```python
from build123d import *

# Parameters (mm, degrees)
PAD006_DEPTH    = 5.1
PAD007_DEPTH    = 2
SKETCH012_W     = 19.5
SKETCH012_H     = 3.5
POCKET004_DEPTH = 26
POCKET005_DEPTH = 5
SKETCH014_R     = 0.575
POCKET006_DEPTH = 3.6
SKETCH015_R     = 1
POCKET007_DEPTH = 2
SKETCH016_W     = 4.5
SKETCH016_H     = 1
PAD008_DEPTH    = 1
CHAMFER_SIZE    = 0.99
SKETCH017_W     = 4.5
SKETCH017_H     = 1
PAD009_DEPTH    = 1
CHAMFER001_SIZE = 0.99
SKETCH018_W     = 9.5
SKETCH018_H     = 10
POCKET008_DEPTH = 4.4
SKETCH022_W     = 4.5
SKETCH022_H     = 1
PAD011_DEPTH    = 1
CHAMFER002_SIZE = 0.99
SKETCH023_W     = 10
SKETCH023_H     = 23.75
PAD012_DEPTH    = 5.1


with BuildPart() as part:
    # Sketch010 → Pad006 (new body)
    with BuildSketch(Plane.XY.offset(7.4)):
        with BuildLine():
            Line((149.259997, 103.29), (149.259997, 4))
            ThreePointArc((145.259999, 0), (148.088425, 1.171573), (149.259997, 4))
            Line((3.999999, 0), (145.259999, 0))
            ThreePointArc((0, 4), (1.171572, 1.171573), (3.999999, 0))
            Line((0, 103.29), (0, 4))
            ThreePointArc((3.999997, 107.29), (1.171572, 106.118426), (0, 103.29))
            Line((3.999997, 107.29), (145.259997, 107.29))
            ThreePointArc((149.259997, 103.29), (148.088425, 106.118427), (145.259997, 107.29))
        make_face()
        with BuildLine():
            Line((3.999997, 105.69), (145.259997, 105.69))
            ThreePointArc((147.659997, 103.29), (146.957054, 104.987056), (145.259997, 105.69))
            Line((147.659997, 103.29), (147.659997, 4))
            ThreePointArc((145.259999, 1.6), (146.957054, 2.302944), (147.659997, 4))
            Line((66.05, 1.6), (145.259999, 1.6))
            Line((66.05, 1.6), (66.05, 25.35))
            Line((66.05, 25.35), (38.05, 25.35))
            Line((38.05, 25.35), (38.05, 1.6))
            Line((4, 1.6), (38.05, 1.6))
            ThreePointArc((1.6, 4), (2.302944, 2.302944), (4, 1.6))
            Line((1.6, 103.29), (1.6, 4))
            ThreePointArc((3.999997, 105.69), (2.302943, 104.987055), (1.6, 103.29))
        make_face(mode=Mode.SUBTRACT)
    extrude(amount=PAD006_DEPTH)

    # Sketch011 (on Face22 of Pad006) → Pad007 (join)
    with BuildSketch(Plane.XY.offset(12.5)):
        with BuildLine():
            Line((149.259997, 103.29), (149.259997, 4))
            ThreePointArc((145.259999, 0), (148.088425, 1.171573), (149.259997, 4))
            Line((3.999999, 0), (145.259999, 0))
            ThreePointArc((0, 4), (1.171572, 1.171573), (3.999999, 0))
            Line((0, 103.29), (0, 4))
            ThreePointArc((3.999997, 107.29), (1.171572, 106.118426), (0, 103.29))
            Line((3.999997, 107.29), (145.259997, 107.29))
            ThreePointArc((149.259997, 103.29), (148.088425, 106.118427), (145.259997, 107.29))
        make_face()
        Polygon((8.05, 102.19), (8.05, 7.1), (28.05, 7.1), (28.05, 25.35), (66.05, 25.35), (66.05, 7.1), (141.209997, 7.1), (141.209997, 83.13), (122.759997, 83.13), (122.759997, 102.19), align=None, mode=Mode.SUBTRACT)
    extrude(amount=PAD007_DEPTH)

    # Sketch012 (on Face26 of Pad007) → Pocket004 (cut)
    with BuildSketch(Plane.YZ.offset(66.05)):
        with Locations((13.3, 9.15)):
            Rectangle(SKETCH012_W, SKETCH012_H)
    extrude(amount=-POCKET004_DEPTH, mode=Mode.SUBTRACT)

    # Sketch013 (on Face25 of Pocket004) → Pocket005 (cut)
    with BuildSketch(Plane.XY.offset(14.5)):
        with BuildLine():
            ThreePointArc((45.3, 15.325), (42.8, 12.825), (45.3, 10.325))
            Line((45.3, 10.325), (46.8, 10.325))
            ThreePointArc((46.8, 10.325), (49.3, 12.825), (46.8, 15.325))
            Line((45.3, 15.325), (46.8, 15.325))
        make_face()
    extrude(amount=-POCKET005_DEPTH, mode=Mode.SUBTRACT)

    # Sketch014 (on Face29 of Pocket005) → Pocket006 (cut)
    with BuildSketch(Plane(origin=(0, 0, 10.9), x_dir=(1, 0, 0), z_dir=(0, 0, -1))):
        with Locations((56.8, -7.825)):
            Circle(SKETCH014_R)
        with Locations((56.8, -17.825)):
            Circle(SKETCH014_R)
    extrude(amount=-POCKET006_DEPTH, mode=Mode.SUBTRACT)

    # Sketch015 (on Face29 of Pocket006) → Pocket007 (cut)
    with BuildSketch(Plane(origin=(0, 0, 10.9), x_dir=(1, 0, 0), z_dir=(0, 0, -1))):
        with Locations((56.8, -17.825)):
            Circle(SKETCH015_R)
        with Locations((56.8, -7.825)):
            Circle(SKETCH015_R)
    extrude(amount=-POCKET007_DEPTH, mode=Mode.SUBTRACT)

    # Sketch016 (on Face6 of Pocket007) → Pad008 (join)
    with BuildSketch(Plane.YZ.offset(147.659997)):
        with Locations((11.3, 7.9)):
            Rectangle(SKETCH016_W, SKETCH016_H)
        with Locations((95.99, 7.9)):
            Rectangle(SKETCH016_W, SKETCH016_H)
    extrude(amount=-PAD008_DEPTH)

    # Chamfer
    chamfer_edges = [part.edges().sort_by_distance(p)[0] for p in [
        (146.659997, 11.3, 7.4),
        (146.659997, 95.99, 7.4),
    ]]
    chamfer(chamfer_edges, length=CHAMFER_SIZE)

    # Sketch017 (on Face31 of Chamfer) → Pad009 (join)
    with BuildSketch(Plane(origin=(1.6, 0, 0), x_dir=(0, -1, 0), z_dir=(-1, 0, 0))):
        with Locations((-95.99, 7.9)):
            Rectangle(SKETCH017_W, SKETCH017_H)
        with Locations((-11.3, 7.9)):
            Rectangle(SKETCH017_W, SKETCH017_H)
    extrude(amount=-PAD009_DEPTH)

    # Chamfer001
    chamfer001_edges = [part.edges().sort_by_distance(p)[0] for p in [
        (2.6, 95.99, 7.4),
        (2.6, 11.3, 7.4),
    ]]
    chamfer(chamfer001_edges, length=CHAMFER001_SIZE)

    # Sketch018 (on Face47 of Chamfer001) → Pocket008 (cut)
    with BuildSketch(Plane.XY.offset(14.5)):
        with Locations((133.009997, 102.29)):
            Rectangle(SKETCH018_W, SKETCH018_H)
    extrude(amount=-POCKET008_DEPTH, mode=Mode.SUBTRACT)

    # Sketch022 (on Face31 of Pocket008) → Pad011 (join)
    with BuildSketch(Plane(origin=(0, 105.69, 0), x_dir=(-1, 0, 0), z_dir=(0, 1, 0))):
        with Locations((-111.959997, 7.9)):
            Rectangle(SKETCH022_W, SKETCH022_H)
    extrude(amount=-PAD011_DEPTH)

    # Chamfer002
    chamfer002_edges = [part.edges().sort_by_distance(p)[0] for p in [
        (111.959997, 104.69, 7.4),
    ]]
    chamfer(chamfer002_edges, length=CHAMFER002_SIZE)

    # Sketch023 (on Face42 of Chamfer002) → Pad012 (join)
    with BuildSketch(Plane(origin=(0, 0, 12.5), x_dir=(1, 0, 0), z_dir=(0, 0, -1))):
        with Locations((33.05, -13.475)):
            Rectangle(SKETCH023_W, SKETCH023_H)
    extrude(amount=PAD012_DEPTH)


solid = part.part
```
For this review, take the finished solid that the model builds, in its own axes (mm). A direction names the side the tool comes from. Round coordinates to 2 decimals unless told otherwise and drop trailing zeros. Write each loop counter-clockwise with the first axis right and the second up, starting at its lowest first coordinate (ties: lowest second). Pieces come first, ordered by that corner, then holes. Notation, with made-up numbers: (60.5, 64.5) -> (98.5, 64.5) arc R8 ccw to (98.5, 79.5) -> close; hole circle Ø3 at (-8, -3). An arc over 180 degrees is marked (long way). One line per question, with ' | ' between items. Start each with the question number.
1) Add section D-D (x = 63.5). Write out the cut boundary in (y, z).
2) For pin 1 Ø1.1 at (y, z) = (105, 8) entering from +X; pin 2 Ø0.5 at (x, z) = (147.5, 8) entering from +Y; pin 3 Ø0.6 at (x, y) = (56.5, 18) entering from -Z, all flat-tipped, find the tip position at first contact; note any pin that passes through.
3) Add section B-B (y = 86). Write out the cut boundary in (x, z).
4) Add section C-C (x = 34.5). Write out the cut boundary in (y, z), and give its area (3 significant figures).
5) Mouldability with a two-part tool opening along X and no side actions: class faces 1 (the cylindrical face through (1.141, 1.203, 10.9)), 2 (the flat face through (53, 3.55, 9)), 3 (the flat face through (64, 22, 14.5)), 4 (the cylindrical face through (148.057, 1.141, 10.9)) as +X half, -X half, draft (parallel to the pull), parting line (faces both ways), or undercut.
6) Wall thickness on line 1 along Y through (x, z) = (56.8, 11.9) (3 decimals); line 2 along X through (y, z) = (10, 11.5); line 3 along Y through (x, z) = (46.5, 10.25): over which ranges is each line inside the solid? List them lowest first.
7) Machinability: for faces 5 (the flat face through (53, 23.05, 9)), 6 (the cylindrical face through (1.203, 106.149, 10.9)), 7 (the flat face through (47, 25.35, 11)), which of the approach directions +Z, -Z, +X, -X, +Y, -Y give a long, thin tool a straight path to every point of the face, cutting with its end or side? Answer none if there is none.
8) Add section A-A (x = 13). Write out the cut boundary in (y, z).
Reported:
1) outline: (0, 7.4) -> (3.55, 7.4) -> (3.55, 10.9) -> (23.05, 10.9) -> (23.05, 7.4) -> (25.35, 7.4) -> (25.35, 14.5) -> (0, 14.5) -> close; (102.19, 12.5) -> (105.69, 12.5) -> (105.69, 7.4) -> (107.29, 7.4) -> (107.29, 14.5) -> (102.19, 14.5) -> close
2) pin 1: stops at x = 149.09 | pin 2: stops at y = 106.76 | pin 3: stops at z = 12.9
3) outline: (0, 7.4) -> (1.6, 7.4) -> (1.6, 12.5) -> (8.05, 12.5) -> (8.05, 14.5) -> (0, 14.5) -> close; (122.76, 12.5) -> (147.66, 12.5) -> (147.66, 7.4) -> (149.26, 7.4) -> (149.26, 14.5) -> (122.76, 14.5) -> close
4) outline: (0, 7.4) -> (25.35, 7.4) -> (25.35, 14.5) -> (0, 14.5) -> close; (102.19, 12.5) -> (105.69, 12.5) -> (105.69, 7.4) -> (107.29, 7.4) -> (107.29, 14.5) -> (102.19, 14.5) -> close | area: 198 mm²
5) face 1: -X half | face 2: undercut | face 3: draft | face 4: +X half
6) line 1: y = 0 to 6.825, 8.825 to 16.825, 18.825 to 25.35, 105.69 to 107.29 | line 2: x = 0 to 1.6, 28.05 to 66.05, 147.66 to 149.26 | line 3: y = 0 to 3.55, 23.05 to 25.35, 105.69 to 107.29
7) face 5: -Z | face 6: +Z, -Z, -X, +Y | face 7: +Z, -Z
8) outline: (0, 7.4) -> (1.6, 7.4) -> (1.6, 12.5) -> (7.1, 12.5) -> (7.1, 14.5) -> (0, 14.5) -> close; (102.19, 12.5) -> (105.69, 12.5) -> (105.69, 7.4) -> (107.29, 7.4) -> (107.29, 14.5) -> (102.19, 14.5) -> close
